Input: part model. Units: mm. Frame: model coordinates. A direction names the side the tool comes from. Give positions to 0.01 mm unless a question says otherwise; leave off trailing zeros. Loops run counter-clockwise (first coordinate to the right, second up) from the corner with the lowest first, then second, coordinate; pieces in that order, holes last.
from build123d import *

# Parameters (mm, degrees)
CYLINDER017_R     = 1.9
CYLINDER017_DEPTH = 8
CYLINDER022_R     = 2.5
CYLINDER022_DEPTH = 5
PRISM_DEPTH       = 15


with BuildPart() as zylinder017:
    # Cylinder017 → Cylinder017 (new body)
    with BuildSketch(Plane.XY):
        Circle(CYLINDER017_R)
    extrude(amount=CYLINDER017_DEPTH)


with BuildPart() as zylinder020:
    # Cylinder022 → Cylinder022 (new body)
    with BuildSketch(Plane.XY.offset(10)):
        Circle(CYLINDER022_R)
    extrude(amount=CYLINDER022_DEPTH)


with BuildPart() as shaft_fixer:
    # Prism → Prism (new body)
    with BuildSketch(Plane.XY):
        Polygon((5.47476, 0), (2.73738, 4.741281), (-2.73738, 4.741281), (-5.47476, 0), (-2.73738, -4.741281), (2.73738, -4.741281), align=None)
    extrude(amount=PRISM_DEPTH)

    # Cut039: cut Zylinder020
    add(zylinder020.part, mode=Mode.SUBTRACT)

    # Cut040: cut Zylinder017
    add(zylinder017.part, mode=Mode.SUBTRACT)


with BuildPart() as shaft_fixer_1:
    # Cut040 placement: moved
    add(shaft_fixer.part.moved(Location((0, 0, 18))))


solid = shaft_fixer_1.part
(1) Cut plane A-A (z = 28.5). Return the cut outline in (x, y), and give its area (3 significant figures).
Values follow:
outline: (-5.47, 0) - (-2.74, -4.74) - (2.74, -4.74) - (5.47, 0) - (2.74, 4.74) - (-2.74, 4.74) - close; hole circle Ø5 at (0, 0)
area: 58.2 mm2
(2) Ray query, probe 1 along Y at (x, z) = (0, 23.5); probe 2 along Z at (x, y) = (-2, -1); probe 3 along X at (y, z) = (-0.5, 27.5). Return the intervals inside material, ascending.
Values follow:
probe 1: y = -4.74 to -1.9, 1.9 to 4.74
probe 2: z = 18 to 28
probe 3: x = -5.19 to 5.19
(3) Mould query, pull axis Y, two halves, no side actions, for faces 4 (the flat face through (0, 4.741, 25)), 5 (the cylindrical face through (-1.9, 0.08, 21.94)), 6 (the flat face through (-4.125, -2.337, 25.395)), 7 (the flat face through (2.4, 0.1, 18)). Classes: +Y half, -Y half, draft (parallel to the pull), parting line (faces both ways), or undercut.
Values follow:
face 4: +Y half
face 5: undercut
face 6: -Y half
face 7: draft
(4) Reachability of faces 1 (the flat face through (0, 0, 28)), 2 (the flat face through (-3, 0, 33)), 3 (the flat face through (0, 0, 26)) from +Z, -Z, +X, -X, +Y, -Y: full face, straight path, thin tool, end or side. Return the list, or none.
Values follow:
face 1: +Z
face 2: +Z, +X, -X, +Y, -Y
face 3: -Z
(5) Cut plane B-B (x = 0). Return the cut outline in (y, z), and give its area (3 significant figures).
Values follow:
outline: (-4.74, 18) - (-1.9, 18) - (-1.9, 26) - (1.9, 26) - (1.9, 18) - (4.74, 18) - (4.74, 33) - (2.5, 33) - (2.5, 28) - (-2.5, 28) - (-2.5, 33) - (-4.74, 33) - close
area: 86.8 mm2
(6) Cut plane D-D (z = 19.5). Return the cut outline in (x, y), and give its area (3 significant figures).
Values follow:
outline: (-5.47, 0) - (-2.74, -4.74) - (2.74, -4.74) - (5.47, 0) - (2.74, 4.74) - (-2.74, 4.74) - close; hole circle Ø3.8 at (0, 0)
area: 66.5 mm2
(7) Cut plane C-C (y = -1.25). Return the cut outline in (x, z), and give its area (3 significant figures).
Values follow:
outline: (-4.75, 18) - (-1.43, 18) - (-1.43, 26) - (1.43, 26) - (1.43, 18) - (4.75, 18) - (4.75, 33) - (2.17, 33) - (2.17, 28) - (-2.17, 28) - (-2.17, 33) - (-4.75, 33) - close
area: 98.0 mm2
(8) Pin query (flat end, axial travel): pin 1 Ø3.5 at (x, y) = (0, 0) entering from +Z; pin 2 Ø3 at (y, z) = (0.5, 31) entering from -X; pin 3 Ø1.1 at (x, y) = (-1, -0.5) entering from -Z. Return the tip coordinate at first contact, or that it passes through.
Values follow:
pin 1: stops at z = 28
pin 2: stops at x = -5.47
pin 3: stops at z = 26
